Read the model definition and answer for the solid it produces. Units are mm, in the model's axes. A direction names the side the tool comes from. Coordinates: 2 decimals unless noted, no trailing zeros. Order: outer loops, then holes, each group sorted by start corner. A loop starts at its lowest first (then second) coordinate and runs counter-clockwise, first axis right, second up. Notation, with made-up numbers: (-25.75, 26) - (18.25, 26) arc R19 ccw to (18.25, 49) - close; hole circle Ø5 at (-26, -18). An arc over 180 degrees is marked (long way). Answer as a JSON object with one key per item and string values. Group by question number.
Autodesk Inventor part; units mm, degrees
ref_plane "YZ Plane" through (0, 0, 0) normal (1, 0, 0) x (0, 1, 0)
ref_plane "XZ Plane" through (0, 0, 0) normal (0, 1, 0) x (-1, 0, 0)
ref_plane "XY Plane" through (0, 0, 0) normal (0, 0, 1) x (1, 0, 0)
sketch "Sketch1" plane through (0, 0, 0) normal (1, 0, 0) x (0, 1, 0)
  circle A0 centre (0, 0) radius 2.7
  line L0 (-1.85, -2.7) -> (1.85, -2.7)
  line L1 (1.85, -2.7) -> (1.85, 2.7)
  line L2 (1.85, 2.7) -> (-1.85, 2.7)
  line L3 (-1.85, 2.7) -> (-1.85, -2.7)
  line L4 (-1.85, -2.7) -> (1.85, 2.7) construction
  line L5 (1.85, -2.7) -> (-1.85, 2.7) construction
  point P0 (-1.85, 1.9666)
  point P1 (-1.85, -1.9666)
  point P2 (1.85, -1.9666)
  point P3 (1.85, 1.9666)
  dimension "d0" = 5.4
  dimension "d1" = 3.7
  dimension "d2" = 5.4
extrude "Extrusion1" add sketch "Sketch1" against normal blind 70 contours L1 A0 L3
sketch "Sketch2" plane through (0, 0, 0) normal (1, 0, 0) x (0, 0, -1)
  circle A0 centre (0, 0) radius 4
extrude "Extrusion2" add sketch "Sketch2" along normal blind 2
properties part number "Axle_3DPrint"
1. Given pin 1 (3 mm diameter, centred on x = -26, y = 2.5, fed in from -Z); pin 2 (1.2 mm diameter, centred on x = -34, z = -1, fed in from -Y); pin 3 (3 mm diameter, centred on x = -59.5, y = 0, fed in from +Z), each flat-ended and moving along its own axis, determine where each tip first touches the part or whether it passes through.
2. A cutting plane is placed at B-B on z = 0. Write down the section's boundary in (x, y).
3. A cutting plane is placed at C-C on x = -16.5. Write down the section's boundary in (y, z), and give its area (3 significant figures).
4. A cutting plane is placed at A-A on y = 0. Write down the section's boundary in (x, z), and give its area (3 significant figures).
5. A cutting plane is placed at D-D on y = -3. Write down the section's boundary in (x, z), and give its area (3 significant figures).
6. Straight lines are drawn through the part: L1, parallel to X at y = 0.25, z = 3.25; L2, parallel to Y at x = -60, z = 0.25; L3, parallel to Z at x = -30, y = -0.25. For each, find the intervals that lie inside material, in ascending order.
7. For faces 1 (the flat face through (0, -3, 0)), 2 (the cylindrical face through (-34.5, 0, -2.7)), 3 (the cylindrical face through (-34.5, 0, 2.7)), determine the directions among +Z, -Z, +X, -X, +Y, -Y from which every point of the face is accessible in a straight line to the end or side of a thin tool.
Derived:
{
 "1": {"pin 1": "stops at z = -2.51", "pin 2": "stops at y = -1.85", "pin 3": "stops at z = 2.7"},
 "2": {"outline": "(-70, -1.85) - (0, -1.85) - (0, -4) - (2, -4) - (2, 4) - (0, 4) - (0, 1.85) - (-70, 1.85) - close"},
 "3": {"outline": "(-1.85, -1.97) arc R2.7 ccw to (1.85, -1.97) - (1.85, 1.97) arc R2.7 ccw to (-1.85, 1.97) - close", "area": "18.3 mm2"},
 "4": {"outline": "(-70, -2.7) - (0, -2.7) - (0, -4) - (2, -4) - (2, 4) - (0, 4) - (0, 2.7) - (-70, 2.7) - close", "area": "394 mm2"},
 "5": {"outline": "(0, -2.65) - (2, -2.65) - (2, 2.65) - (0, 2.65) - close", "area": "10.6 mm2"},
 "6": {"L1": "x = 0 to 2", "L2": "y = -1.85 to 1.85", "L3": "z = -2.69 to 2.69"},
 "7": {"face 1": "-X", "face 2": "-Z, -X", "face 3": "+Z, -X"}
}
